For this review, use the dimensioned drawing (mm, ordinates from the lowest corner) and the shaded views. A direction names the side the tool comes from. Round coordinates to 2 decimals unless told otherwise and drop trailing zeros. Loops run counter-clockwise (first coordinate to the right, second up) from the corner with the lowest first, then second, coordinate; pieces in that order, holes last. Notation, with made-up numbers: (26, 20) -> (52, 20) arc R17 cw to (52, 26) -> close; hole circle Ø5 at (-8, 9.25). An arc over 180 degrees is marked (long way). Write each question's results on one line, items separated by ' | '.
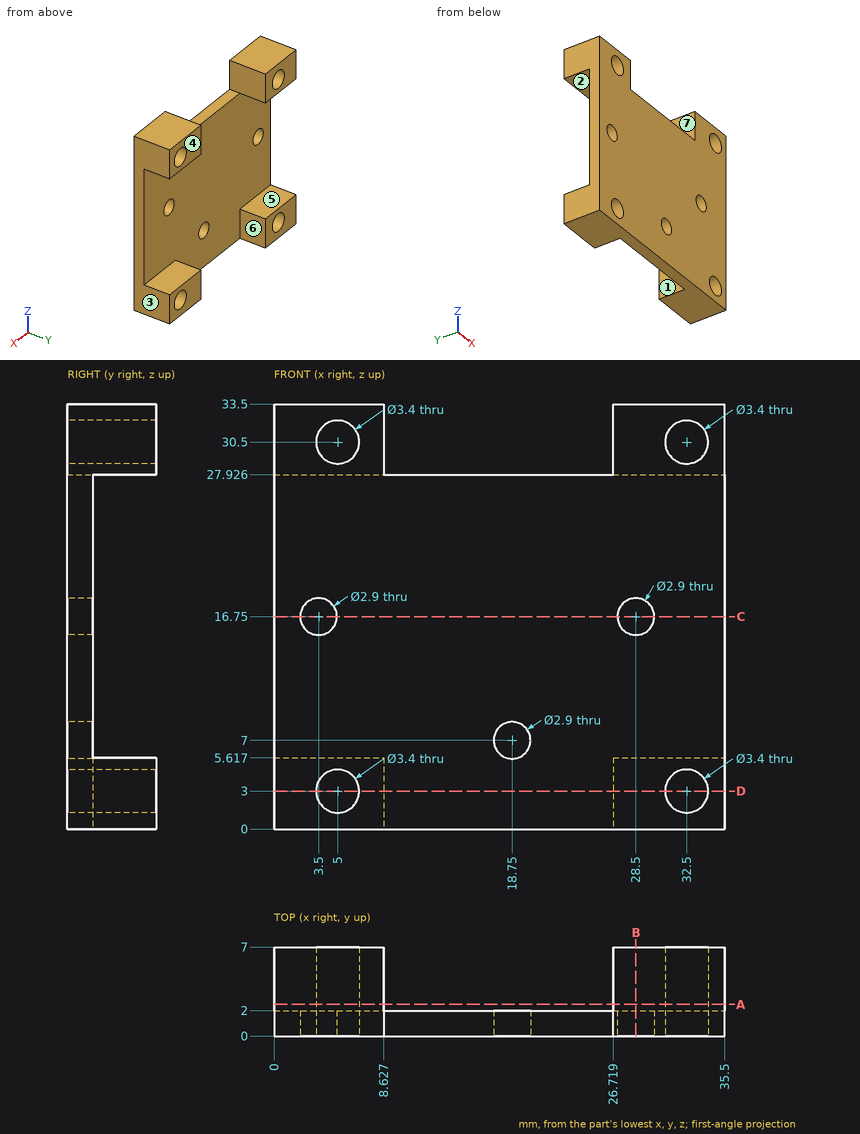
1. For pin 1 (4 mm diameter, centred on x = 9.5, z = 16.5, fed in from +Y); pin 2 (2.5 mm diameter, centred on x = 5, z = 3, fed in from -Y); pin 3 (5.5 mm diameter, centred on x = 32.5, z = 3, fed in from -Y), all flat-tipped, find the tip position at first contact; note any pin that passes through.
Values found:
pin 1: stops at y = 2 | pin 2: passes through | pin 3: stops at y = 0
2. Draft analysis for pull direction X (two halves, no side actions). For the marked faces 1, 2 and 3, state which applies: released by +X, released by -X, zero draft, split by the parting line, or undercut.
Values found:
face 1: undercut | face 2: zero draft | face 3: released by +X
3. Consider section D-D (z = 3). State the section outline as (x, y) points.
Values found:
outline: (0, 0) -> (3.3, 0) -> (3.3, 7) -> (0, 7) -> close; (6.7, 0) -> (30.8, 0) -> (30.8, 7) -> (26.72, 7) -> (26.72, 2) -> (8.63, 2) -> (8.63, 7) -> (6.7, 7) -> close; (34.2, 0) -> (35.5, 0) -> (35.5, 7) -> (34.2, 7) -> close
4. To check wall thickness, follow probe 1 along X at (y, z) = (1.45, 16.75); probe 2 along Z at (x, y) = (27.5, 5.75); probe 3 along X at (y, z) = (6.75, 31) (1 decimal). State the ranges of each line that lie inside material, in increasing order.
Values found:
probe 1: x = 0 to 2.05, 4.95 to 27.05, 29.95 to 35.5 | probe 2: z = 0 to 5.62, 27.93 to 33.5 | probe 3: x = 0 to 3.4, 6.6 to 8.6, 26.7 to 30.9, 34.1 to 35.5
5. Consider section A-A (y = 2.5). State the section outline as (x, z) points.
Values found:
outline: (0, 0) -> (8.63, 0) -> (8.63, 5.62) -> (0, 5.62) -> close; (0, 27.93) -> (8.63, 27.93) -> (8.63, 33.5) -> (0, 33.5) -> close; (26.72, 0) -> (35.5, 0) -> (35.5, 5.62) -> (26.72, 5.62) -> close; (26.72, 27.93) -> (35.5, 27.93) -> (35.5, 33.5) -> (26.72, 33.5) -> close; hole circle Ø3.4 at (5, 3); hole circle Ø3.4 at (5, 30.5); hole circle Ø3.4 at (32.5, 3); hole circle Ø3.4 at (32.5, 30.5)
6. Tool access review of the marked faces 4, 5, 6 and 7: name each direction out of +Z, -Z, +X, -X, +Y, -Y from which nothing blocks a thin tool from reaching the whole face with its end or side.
Values found:
face 4: +Z, -Z, +X, -X, +Y | face 5: +X, -X, +Y | face 6: +Z, -Z, +Y | face 7: +Z, +Y, -Y
7. Consider section C-C (z = 16.75). State the section outline as (x, y) points.
Values found:
outline: (0, 0) -> (2.05, 0) -> (2.05, 2) -> (0, 2) -> close; (4.95, 0) -> (27.05, 0) -> (27.05, 2) -> (4.95, 2) -> close; (29.95, 0) -> (35.5, 0) -> (35.5, 2) -> (29.95, 2) -> close
8. Consider section B-B (x = 28.5). State the section outline as (y, z) points, plus the area to 3 significant figures.
Values found:
outline: (0, 0) -> (7, 0) -> (7, 5.62) -> (2, 5.62) -> (2, 15.3) -> (0, 15.3) -> close; (0, 18.2) -> (2, 18.2) -> (2, 27.93) -> (7, 27.93) -> (7, 33.5) -> (0, 33.5) -> close | area: 117 mm2
